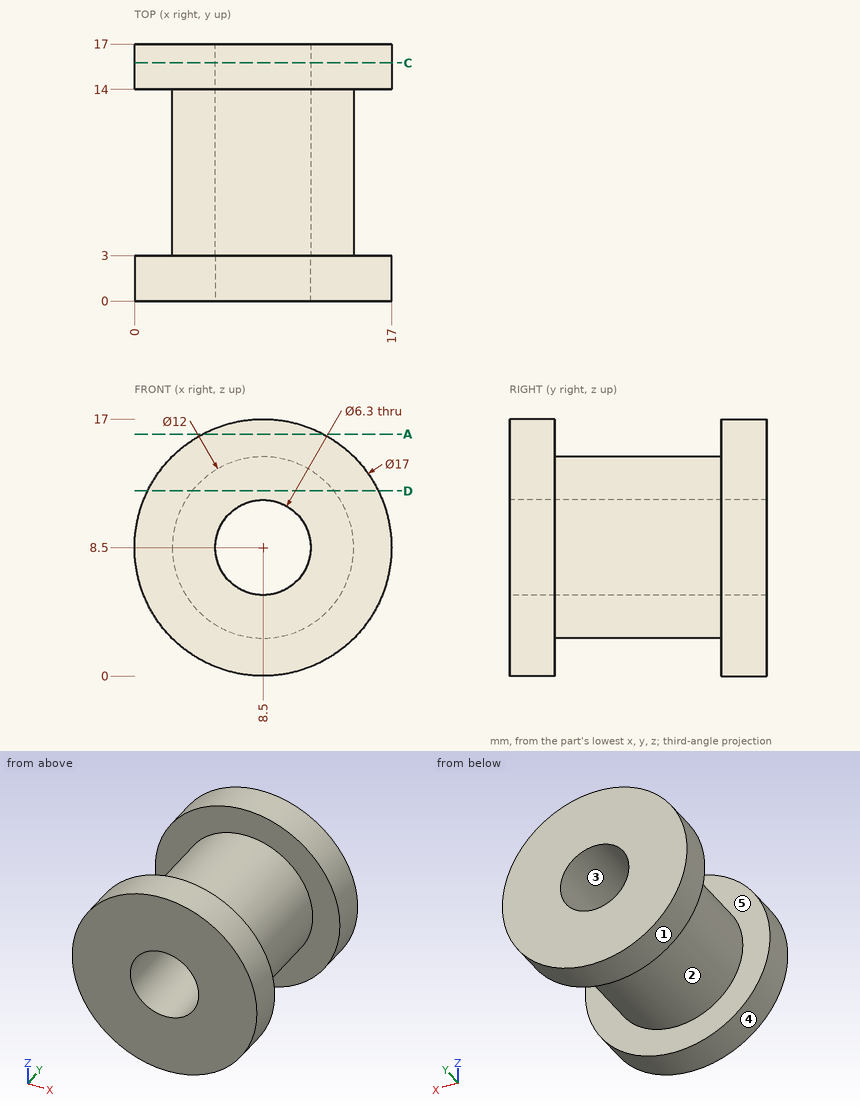
Could you check a few things on this drawing? It's one solid part, dimensions in mm from its lowest x, y, z. A direction names the side the tool comes from. Give positions to 0.01 mm unless a question says otherwise; leave off trailing zeros. Write each loop counter-clockwise with the first axis right and the second up, starting at its lowest first coordinate (ties: lowest second). Pieces come first, ordered by that corner, then holes. Notation, with made-up numbers: (47, 38.25) -> (65, 38.25) arc R17 ccw to (65, 50.25) -> close; hole circle Ø7 at (85, 65). An arc over 180 degrees is marked (long way). Answer as a JSON object with one key per item and string values.
Q1. Which directions (+Z, -Z, +X, -X, +Y, -Y) give clear straight access to the entire face, cutting with the end or side of a thin tool? Please do the marked faces 1 and 2.
Taken from the geometry:
{"face 1": "+Y, -Y", "face 2": "none"}
Q2. We'd pull the mould along Z, two halves only. Please class the marked faces 3, 4 and 5: released by +Z, released by -Z, zero draft, split by the parting line, or undercut.
Taken from the geometry:
{"face 3": "undercut", "face 4": "split by the parting line", "face 5": "zero draft"}
Q3. Suppose I cut it at C-C on y = 15.75. Write out the boundary of the cut face in (x, z).
Taken from the geometry:
{"outline": "circle Ø17 at (8.5, 8.5); hole circle Ø6.3 at (8.5, 8.5)"}
Q4. Please list where these lines run through material, in increasing order: L1, parallel to X at y = 3.5, z = 8.5; L2, parallel to Y at x = 14, z = 11.5.
Taken from the geometry:
{"L1": "x = 2.5 to 5.35, 11.65 to 14.5", "L2": "y = 0 to 3, 14 to 17"}
Q5. Suppose I cut it at D-D on z = 12.25. Write out the boundary of the cut face in (x, y), then the cut area to 3 significant figures.
Taken from the geometry:
{"outline": "(0.87, 0) -> (16.13, 0) -> (16.13, 3) -> (13.18, 3) -> (13.18, 14) -> (16.13, 14) -> (16.13, 17) -> (0.87, 17) -> (0.87, 14) -> (3.82, 14) -> (3.82, 3) -> (0.87, 3) -> close", "area": "195 mm²"}
Q6. Suppose I cut it at A-A on z = 16. Write out the boundary of the cut face in (x, y), then the cut area to 3 significant figures.
Taken from the geometry:
{"outline": "(4.5, 0) -> (12.5, 0) -> (12.5, 3) -> (4.5, 3) -> close; (4.5, 14) -> (12.5, 14) -> (12.5, 17) -> (4.5, 17) -> close", "area": "48.0 mm²"}
Q7. Will these pins go through, and if not, where does the flat tip stop? pin 1 Ø1 at (x, z) = (14.5, 12.5) entering from -Y; pin 2 Ø2 at (y, z) = (8.5, 7) entering from +X; pin 3 Ø4 at (x, z) = (8.5, 8.5) entering from -Y; pin 4 Ø1.5 at (x, y) = (13, 9) entering from -Z.
Taken from the geometry:
{"pin 1": "stops at y = 0", "pin 2": "stops at x = 14.48", "pin 3": "passes through", "pin 4": "stops at z = 3.82"}
